```python
from build123d import *

# Parameters (mm, degrees)
BOSS_EXTRUDE1_DEPTH = 26
SKETCH2_R           = 1.7
CUT_EXTRUDE1_DEPTH  = 31
CUT_EXTRUDE2_DEPTH  = 1


with BuildPart() as part:
    # Sketch1 → Boss-Extrude1 (new body)
    with BuildSketch(Plane(origin=(0, 0, 0), x_dir=(1, 0, 0), z_dir=(0, 1, 0))):
        with BuildLine():
            Line((-46.998275301, 32.528571429), (-46.998275301, -39.471428571))
            Line((-46.998275301, -39.471428571), (-16.998275301, -39.471428571))
            Line((-16.998275301, -39.471428571), (-16.998275301, -27.971428571))
            ThreePointArc((-16.998275301, -27.971428571), (-41.498275301, -3.471428571), (-16.998275301, 21.028571429))
            Line((-16.998275301, 21.028571429), (-16.998275301, 32.528571429))
            Line((-16.998275301, 32.528571429), (-46.998275301, 32.528571429))
        make_face()
    extrude(amount=BOSS_EXTRUDE1_DEPTH)

    # Sketch2 → Cut-Extrude1 (cut, through all)
    with BuildSketch(Plane(origin=(-16.998275301, 0, 0), x_dir=(0, 0, -1), z_dir=(1, 0, 0))):
        with Locations((-34.471428571, 13)):
            Circle(SKETCH2_R)
        with Locations((27.528571429, 13)):
            Circle(SKETCH2_R)
    extrude(amount=-CUT_EXTRUDE1_DEPTH, mode=Mode.SUBTRACT)

    # Sketch3 → Cut-Extrude2 (cut)
    with BuildSketch(Plane(origin=(-16.998275301, 0, 0), x_dir=(0, 0, -1), z_dir=(1, 0, 0))):
        Polygon((-34.164231178, 21.664809495), (-32.617436306, 21.664809495), (-32.617436306, 21.33916847), (-33.87929528, 21.33916847), (-33.87929528, 20.362245393), (-32.617436306, 20.362245393), (-32.617436306, 20.036604367), (-33.87929528, 20.036604367), (-33.87929528, 18.489809495), (-34.164231178, 18.489809495), align=None)
        with BuildLine():
            Line((-30.337949127, 21.664809495), (-30.337949127, 21.33916847))
            Line((-30.337949127, 21.33916847), (-31.417271042, 21.33916847))
            Line((-31.417271042, 21.33916847), (-31.588995801, 20.504077324))
            add(Edge.make_bspline(
                [(-31.588995801, 20.504077324), (-31.555380829, 20.513357642), (-31.490257138, 20.53133679), (-31.394136407, 20.551299168), (-31.302884908, 20.563332821), (-31.243670822, 20.564975938), (-31.215017436, 20.565771034)],
                knots=[0, 0, 0, 0, 0.000104595, 0.000202637, 0.000294305, 0.000380252, 0.000380252, 0.000380252, 0.000380252], degree=3))
            add(Edge.make_bspline(
                [(-31.215017436, 20.565771034), (-31.179562901, 20.565003649), (-31.109850426, 20.56349478), (-31.007852238, 20.54900603), (-30.910485971, 20.526200536), (-30.817955249, 20.494341206), (-30.730088893, 20.453601662), (-30.647695319, 20.402711002), (-30.569537784, 20.343262909), (-30.497018431, 20.27491422), (-30.431228522, 20.199692467), (-30.37338366, 20.118813541), (-30.324250453, 20.033063448), (-30.284734626, 19.941622896), (-30.253180265, 19.845502806), (-30.232178099, 19.743691821), (-30.218192941, 19.637149598), (-30.216630491, 19.564301881), (-30.215833742, 19.527154247)],
                knots=[0, 0, 0, 0, 0.000106308, 0.000209029, 0.000308378, 0.000405929, 0.000502102, 0.000598312, 0.00069588, 0.000796219, 0.000896736, 0.000995218, 0.001094066, 0.001192613, 0.001293582, 0.001396995, 0.001504047, 0.001615439, 0.001615439, 0.001615439, 0.001615439], degree=3))
            add(Edge.make_bspline(
                [(-30.215833742, 19.527154247), (-30.21643706, 19.501280519), (-30.217635543, 19.449882723), (-30.223730262, 19.373551912), (-30.235464805, 19.298837056), (-30.251219812, 19.225728244), (-30.271669005, 19.154363885), (-30.296424075, 19.084539713), (-30.326719043, 19.01669032), (-30.359948934, 18.950173711), (-30.397365381, 18.886493637), (-30.438893027, 18.826940628), (-30.482767437, 18.770621315), (-30.529976408, 18.718139715), (-30.58095874, 18.669840691), (-30.635096995, 18.625437607), (-30.691959176, 18.584179543), (-30.752425003, 18.547741252), (-30.815147113, 18.51421057), (-30.881031281, 18.48670279), (-30.948577774, 18.462109668), (-31.018758768, 18.44250674), (-31.091415298, 18.427146494), (-31.16666713, 18.416713806), (-31.244119595, 18.409115181), (-31.296620499, 18.408639514), (-31.323140433, 18.408399239)],
                knots=[0, 0, 0, 0, 7.7636e-05, 0.000154223, 0.000229512, 0.000304362, 0.000378447, 0.000452077, 0.000526407, 0.000601214, 0.00067506, 0.000747747, 0.00081887, 0.000889121, 0.000959302, 0.001029336, 0.001099058, 0.00116985, 0.001240974, 0.00131221, 0.00138383, 0.001456517, 0.001530612, 0.001606437, 0.001684346, 0.001763871, 0.001763871, 0.001763871, 0.001763871], degree=3))
            add(Edge.make_bspline(
                [(-31.323140433, 18.408399239), (-31.354776297, 18.409025928), (-31.417016122, 18.410258864), (-31.508202636, 18.423157061), (-31.5959366, 18.441630042), (-31.679511763, 18.469421516), (-31.759677124, 18.504244276), (-31.835353446, 18.548255374), (-31.9084744, 18.598129276), (-31.976067462, 18.656985024), (-32.038801936, 18.721315679), (-32.094959984, 18.791127253), (-32.144974014, 18.865267533), (-32.188043113, 18.944096573), (-32.224780604, 19.02740724), (-32.253641343, 19.115511677), (-32.276935279, 19.207949537), (-32.286789954, 19.271588793), (-32.29179528, 19.303912059)],
                knots=[0, 0, 0, 0, 9.4843e-05, 0.000186593, 0.000275792, 0.000363484, 0.000450342, 0.000537514, 0.000625728, 0.000715478, 0.000805885, 0.000894984, 0.00098389, 0.001073836, 0.001164117, 0.001256635, 0.001351658, 0.001449737, 0.001449737, 0.001449737, 0.001449737], degree=3))
            Line((-32.29179528, 19.303912059), (-32.006859383, 19.303912059))
            add(Edge.make_bspline(
                [(-32.006859383, 19.303912059), (-31.999848477, 19.273634849), (-31.986373127, 19.215440369), (-31.956795055, 19.133678367), (-31.920631011, 19.060817357), (-31.877628495, 18.995893521), (-31.826329539, 18.939279645), (-31.767792128, 18.888827024), (-31.702162408, 18.843311014), (-31.629234264, 18.805371789), (-31.552296685, 18.773015134), (-31.471772144, 18.751468954), (-31.389853202, 18.736318858), (-31.334446394, 18.734802333), (-31.306603974, 18.734040265)],
                knots=[0, 0, 0, 0, 9.3172e-05, 0.000179081, 0.000260145, 0.000336703, 0.000411917, 0.000488562, 0.000568128, 0.000650923, 0.00073478, 0.000817953, 0.000900557, 0.000983994, 0.000983994, 0.000983994, 0.000983994], degree=3))
            add(Edge.make_bspline(
                [(-31.306603974, 18.734040265), (-31.279427385, 18.734784827), (-31.22591646, 18.736250878), (-31.14716613, 18.747534839), (-31.07113588, 18.764913493), (-30.998575921, 18.790921147), (-30.928216524, 18.822530284), (-30.861837461, 18.863093246), (-30.797518422, 18.909774834), (-30.737258616, 18.96325692), (-30.682068544, 19.022193714), (-30.633304062, 19.085219635), (-30.592685005, 19.152454203), (-30.558454778, 19.222733421), (-30.532462142, 19.29682754), (-30.513919252, 19.374389321), (-30.503030763, 19.455610338), (-30.501532907, 19.511008927), (-30.500769639, 19.539238582)],
                knots=[0, 0, 0, 0, 8.15e-05, 0.000160473, 0.000238226, 0.000315066, 0.000391338, 0.000469218, 0.000547964, 0.000629516, 0.000710512, 0.000789892, 0.000868102, 0.000945761, 0.001024012, 0.00110315, 0.001184644, 0.001269321, 0.001269321, 0.001269321, 0.001269321], degree=3))
            add(Edge.make_bspline(
                [(-30.500769639, 19.539238582), (-30.501366974, 19.564707299), (-30.502536172, 19.61455869), (-30.512088904, 19.687492256), (-30.528705015, 19.756501373), (-30.551768106, 19.821919285), (-30.581050231, 19.883807694), (-30.616833671, 19.94223047), (-30.659789968, 19.99641759), (-30.708859038, 20.046394406), (-30.762614547, 20.092517971), (-30.82198137, 20.13183725), (-30.885717161, 20.164915232), (-30.953054012, 20.193461202), (-31.025593599, 20.213963307), (-31.101899401, 20.229355603), (-31.182795415, 20.238259539), (-31.238104539, 20.239494967), (-31.266534864, 20.240130008)],
                knots=[0, 0, 0, 0, 7.6388e-05, 0.000149519, 0.000220172, 0.000288967, 0.000357247, 0.000425206, 0.000494043, 0.000564207, 0.000635056, 0.000706145, 0.000777268, 0.000850264, 0.000925136, 0.001002969, 0.001083601, 0.001168886, 0.001168886, 0.001168886, 0.001168886], degree=3))
            add(Edge.make_bspline(
                [(-31.266534864, 20.240130008), (-31.291144678, 20.239603329), (-31.3419577, 20.23851587), (-31.419901979, 20.230508977), (-31.50180947, 20.217591903), (-31.587366191, 20.199824378), (-31.676829081, 20.17657333), (-31.770009344, 20.14871089), (-31.8671029, 20.115398791), (-31.932523979, 20.090241712), (-31.966154255, 20.077309495)],
                knots=[0, 0, 0, 0, 7.3822e-05, 0.000152423, 0.000234822, 0.000322511, 0.00041445, 0.000512043, 0.000614219, 0.000722306, 0.000722306, 0.000722306, 0.000722306], degree=3))
            Line((-31.966154255, 20.077309495), (-31.640513229, 21.664809495))
            Line((-31.640513229, 21.664809495), (-30.337949127, 21.664809495))
        make_face()
    extrude(amount=-CUT_EXTRUDE2_DEPTH, mode=Mode.SUBTRACT)


solid = part.part
```
Geometry: final body of the model. Coordinates: model frame, mm. Coordinates: 2 decimals unless noted, no trailing zeros. Order: outer loops, then holes, each group sorted by start corner. A loop starts at its lowest first (then second) coordinate and runs counter-clockwise, first axis right, second up.
Item 1: Section query A-A (y = 13). Output: boundary loops of the cut face in (x, z).
Answer:
outline: (-47, -32.53) - (-17, -32.53) - (-17, -29.23) - (-47, -29.23) - close; (-47, -25.83) - (-17, -25.83) - (-17, -21.03) arc R24.5 cw to (-17, 27.97) - (-17, 32.77) - (-47, 32.77) - close; (-47, 36.17) - (-17, 36.17) - (-17, 39.47) - (-47, 39.47) - close
Item 2: Section query D-D (x = -22). Output: boundary loops of the cut face in (y, z).
Answer:
outline: (0, -32.53) - (26, -32.53) - (26, -20.51) - (0, -20.51) - close; (0, 27.46) - (26, 27.46) - (26, 39.47) - (0, 39.47) - close; hole circle Ø3.4 at (13, -27.53); hole circle Ø3.4 at (13, 34.47)
Item 3: Material intervals for line 1 along Z through (x, y) = (-36, 8.75); line 2 along Z through (x, y) = (-32.5, 9.25); line 3 along X through (y, z) = (13.75, 3), sorted ascending.
Answer:
line 1: z = -32.53 to -11.99, 18.94 to 39.47
line 2: z = -32.53 to -15.5, 22.44 to 39.47
line 3: x = -47 to -41.49
Item 4: Section query C-C (y = 9). Output: boundary loops of the cut face in (x, z).
Answer:
outline: (-47, -32.53) - (-17, -32.53) - (-17, -21.03) arc R24.5 cw to (-17, 27.97) - (-17, 39.47) - (-47, 39.47) - close
Item 5: Section query B-B (x = -29.5). Output: boundary loops of the cut face in (y, z), then the cut area to 3 significant figures.
Answer:
outline: (0, -32.53) - (26, -32.53) - (26, -17.6) - (0, -17.6) - close; (0, 24.54) - (26, 24.54) - (26, 39.47) - (0, 39.47) - close; hole circle Ø3.4 at (13, -27.53); hole circle Ø3.4 at (13, 34.47)
area: 758 mm2
Item 6: Draft query along Z for faces 1 (the face through (-17.998, 20.4, 31.1)), 2 (the face through (-41.492, 12.818, 4.01)), 3 (the face through (-42, 0, 3)), 4 (the face through (-32, 13, -32.529)). Return one class per face: released by +Z, released by -Z, zero draft, split by the parting line, or undercut.
Answer:
face 1: undercut
face 2: undercut
face 3: zero draft
face 4: released by -Z
